Model file for the job. Use its own axes, mm. Face numbers are marked on the shaded views. A direction names the side the tool comes from. Round coordinates to 2 decimals unless told otherwise and drop trailing zeros. Loops run counter-clockwise (first coordinate to the right, second up) from the corner with the lowest first, then second, coordinate; pieces in that order, holes last. Notation, with made-up numbers: M -1,56.25 L 11,56.25 A9 cw 11,67.25 Z; hole C -33,-30 d3. An arc over 180 degrees is marked long. Use a Markdown table: item, result. Add a question column.
Q1. Probe line 1 (Z direction, x = 0, y = -2.75); line 2 (X direction, y = 0.75, z = -0.3); line 3 (Y direction, x = 18, z = 2.25). List the from-to ranges inside material, lowest first. Write a range as from..to.
Q2. Cut at C-C (x = -11.5). Give the cut face in (y, z), plus the area to 3 significant figures.
Q3. Cut at B-B (z = 0). Give the cut face in (x, y), plus the area to 3 significant figures.
Q4. Pin check, flat tips, straight feed: pin 1 (0.5 mm diameter, centred on x = 29, y = -1.5, fed in from -Z); pin 2 (2 mm diameter, centred on y = -1.5, z = -0.5, fed in from -X); pin 3 (1.5 mm diameter, centred on x = -8, y = -4, fed in from +Z). Stop position of each tip, or through.
Q5. Mould opens along X. For the marked faces 6, 7 and 8 say: +X half, -X half, draft (parallel to the pull), parting line (faces both ways), or undercut.
Q6. Cut at A-A (y = -5). Give the cut face in (x, z), plus the area to 3 significant figures.
Q7. Tool access for the marked faces 1, 2, 3, 4 and 5: list every direction of +Z, -Z, +X, -X, +Y, -Y with a clear straight run to the whole face (end or side of a thin tool).
Q8. Cut at D-D (x = 3). Give the cut face in (y, z), plus the area to 3 significant figures.
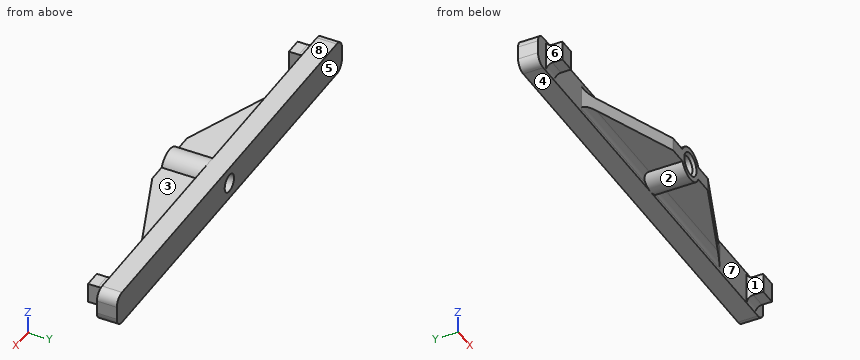
from build123d import *

# Parameters (mm, degrees)
SKETCH1_W                        = 65
SKETCH1_H                        = 5
BODY_DEPTH                       = 3
SKETCH3_W                        = 2.5
SKETCH3_H                        = 3
PEGS_DEPTH                       = 2.5
WEB_DEPTH                        = 1
SKETCH6_R                        = 2.5
HOLE_BOSS_DEPTH                  = 6
M2_5_CLEARANCE_HOLE1_D           = 2.7
M2_5_CLEARANCE_HOLE1_CSINK_D     = 3.5
M2_5_CLEARANCE_HOLE1_CSINK_ANGLE = 90
FILLET1_R                        = 1.5
FILLET2_R                        = 1
FILLET3_R                        = 1


with BuildPart() as part:
    # Sketch1 → body (new body)
    with BuildSketch(Plane(origin=(0, 0, 0), x_dir=(1, 0, 0), z_dir=(0, 1, 0))):
        Rectangle(SKETCH1_W, SKETCH1_H)
    extrude(amount=BODY_DEPTH)

    # Sketch3 → pegs (add)
    with BuildSketch(Plane.XZ):
        with Locations((29, 0)):
            Rectangle(SKETCH3_W, SKETCH3_H)
        with Locations((-29, 0)):
            Rectangle(SKETCH3_W, SKETCH3_H)
    extrude(amount=PEGS_DEPTH)

    # Sketch5 → web (add, symmetric)
    with BuildSketch(Plane.XY):
        Polygon((-20, 0), (20, 0), (5, -6), (-5, -6), align=None)
    extrude(amount=WEB_DEPTH, both=True)

    # Sketch6 → hole-boss (add)
    with BuildSketch(Plane.XZ):
        Circle(SKETCH6_R)
    extrude(amount=HOLE_BOSS_DEPTH)

    # M2.5 Clearance Hole1 (through all)
    with Locations(Plane(origin=(0, -6, 0), x_dir=(-1, 0, 0), z_dir=(0, -1, 0))):
        with Locations((0, 0)):
            CounterSinkHole(M2_5_CLEARANCE_HOLE1_D / 2, M2_5_CLEARANCE_HOLE1_CSINK_D / 2, counter_sink_angle=M2_5_CLEARANCE_HOLE1_CSINK_ANGLE)

    # Fillet1
    fillet1_edges = [part.edges().sort_by_distance(p)[0] for p in [
        (32.5, 1.5, 2.5),
        (-32.5, 1.5, 2.5),
        (-32.5, 1.5, -2.5),
        (32.5, 1.5, -2.5),
    ]]
    fillet(fillet1_edges, radius=FILLET1_R)

    # Fillet2
    fillet2_edges = [part.edges().sort_by_distance(p)[0] for p in [
        (29, 0, 1.5),
        (29, 0, -1.5),
        (-29, 0, 1.5),
        (-29, 0, -1.5),
    ]]
    fillet(fillet2_edges, radius=FILLET2_R - 0.0001)  # a hair under: the kernel refuses the full size

    # Fillet3
    fillet3_edges = [part.edges().sort_by_distance(p)[0] for p in [
        (11.145643924, 0, -1),
        (11.145643924, 0, 1),
        (-11.145643924, 0, -1),
        (-11.145643924, 0, 1),
    ]]
    fillet(fillet3_edges, radius=FILLET3_R)


solid = part.part
Checked values:
| question | item | result |
|---|---|---|
| 1 | line 1 | z = -2.5..-1.35, 1.35..2.5 |
| 1 | line 2 | x = -32.5..-1.32, 1.32..32.5 |
| 1 | line 3 | y = 0..3 |
| 2 | outline | M -3.4,-1 L -1,-1 A1 cw 0,-2 L 0,-2.5 L 3,-2.5 L 3,2.5 L 0,2.5 L 0,2 A1 cw -1,1 L -3.4,1 Z |
| 2 | area | 22.2 mm^2 |
| 3 | outline | M -32.5,0 L -30.25,0 L -30.25,-2.5 L -27.75,-2.5 L -27.75,0 L -20,0 L -5,-6 L -1.75,-6 L -1.35,-5.6 L -1.35,3 L -32.5,3 Z; M 1.35,-5.6 L 1.75,-6 L 5,-6 L 20,0 L 27.75,0 L 27.75,-2.5 L 30.25,-2.5 L 30.25,0 L 32.5,0 L 32.5,3 L 1.35,3 Z |
| 3 | area | 333 mm^2 |
| 4 | pin 1 | stops at z = -1.5 |
| 4 | pin 2 | stops at x = -30.25 |
| 4 | pin 3 | stops at z = 1 |
| 5 | face 6 | -X half |
| 5 | face 7 | undercut |
| 5 | face 8 | draft |
| 6 | outline | M -7.5,-1 L -2.29,-1 A2.5 ccw 2.29,-1 L 7.5,-1 L 7.5,1 L 2.29,1 A2.5 ccw -2.29,1 L -7.5,1 Z; hole C 0,0 d2.7 |
| 6 | area | 34.2 mm^2 |
| 7 | face 1 | +Z, -Z, -Y |
| 7 | face 2 | -Z, -Y |
| 7 | face 3 | +Z, -Y |
| 7 | face 4 | -Z, +X, -X, +Y, -Y |
| 7 | face 5 | +Z, -Z, +X, -X, +Y |
| 8 | outline | M -6,-1 L -1,-1 A1 cw 0,-2 L 0,-2.5 L 3,-2.5 L 3,2.5 L 0,2.5 L 0,2 A1 cw -1,1 L -6,1 Z |
| 8 | area | 27.4 mm^2 |
